Input: part model. Units: mm. Frame: model coordinates. A direction names the side the tool comes from. Coordinates: 2 decimals unless noted, no trailing zeros. Loops run counter-clockwise (first coordinate to the right, second up) from the corner with the lowest first, then second, coordinate; pieces in that order, holes last.
Item 1: Section B-B on x = -115. Return loops of the section in (y, z).
Item 2: Contact query for flat-ended pins moving along their axis: P1, Ø0.5, axis at y = 1, z = -46, coming from the -X side; P2, Ø0.5, axis at x = -48, y = 1, coming from the -Z side; P3, Ø0.8, axis at y = 1, z = -9, coming from the +X side. Output: stop coordinate, or through.
Item 3: Reachability of faces 1 (the flat face through (-176.227, 0.811, -82.597)), 2 (the flat face through (-3.68, 0.81, -83.02)), 3 (the flat face through (-12.056, 0.811, -84.63)), 4 (the flat face through (-91, 1.6, -51)) from +Z, -Z, +X, -X, +Y, -Y: full face, straight path, thin tool, end or side. Return the list, or none.
Item 4: Ray query, line 1 along Z through (x, y) = (-87, 0.6); line 2 along Z through (x, y) = (-103.5, 0.8); line 3 along X through (y, z) = (0.55, -8.5). Return the intervals inside material, ascending.
Item 5: Section D-D on z = -52.5. Return loops of the section in (x, y), and give its area (3 significant figures).
Item 6: Pull-direction query (Z, two-part tool) for faces 5 (the flat face through (-91, 0, -51)), 6 (the flat face through (-175.826, 0.811, -17.954)); classes: released by +Z, released by -Z, zero draft, split by the parting line, or undercut.
Item 7: Section C-C on y = 0.6. Give the number of separate pieces and of enclosed holes in the cut face, and give its area (3 significant figures).
Item 8: Section A-A on z = -109. Return loops of the section in (x, y), and give its area (3 significant figures).
```python
from build123d import *

# Parameters (mm, degrees)
SKETCH1_W           = 80
SKETCH1_H           = 30
SKETCH1_W_2         = 50
BOSS_EXTRUDE1_DEPTH = 1.6
FILLET1_SIZE        = 60
SKETCH6_W           = 80
SKETCH6_H           = 30
CUT_EXTRUDE1_DEPTH  = 10
FILLET3_R           = 20
CUT_EXTRUDE3_REACH  = 256.563
SKETCH9_W           = 15.367
SKETCH9_H           = 16.637
CUT_EXTRUDE5_REACH  = 256.563
SKETCH11_R          = 1.55
SKETCH11_R_2        = 1
SKETCH11_W          = 23.3
SKETCH11_H          = 12.6
CUT_EXTRUDE6_REACH  = 256.563
SKETCH12_W          = 33.087121525
SKETCH12_H          = 10


with BuildPart() as part:
    # Sketch1 → Boss-Extrude1 (new body)
    with BuildSketch(Plane(origin=(0, 0, 0), x_dir=(1, 0, 0), z_dir=(0, 1, 0))):
        with Locations((-90, -15)):
            Rectangle(SKETCH1_W, SKETCH1_H)
        Polygon((0, 180), (-180, 180), (-180, 30), (-130, 30), (-50, 30), (0, 30), align=None)
        with Locations((-25, 15)):
            Rectangle(SKETCH1_W_2, SKETCH1_H)
        with Locations((-155, 15)):
            Rectangle(SKETCH1_W_2, SKETCH1_H)
        with Locations((-90, 15)):
            Rectangle(SKETCH1_W, SKETCH1_H)
    extrude(amount=BOSS_EXTRUDE1_DEPTH)

    # Fillet1
    # a fillet whose section is not a circle: 60 mm, written as the material it takes off along each edge
    with BuildSketch(Plane(origin=(0, -150, -180), x_dir=(0, 0, 1), z_dir=(0, 1, 0)), Plane(origin=(-180, -150, -180), x_dir=(1, 0, 0), z_dir=(0, 1, 0))) as fillet1_piece_1:
        with BuildLine():
            Bezier((FILLET1_SIZE, 0), (0, 0), (0, -FILLET1_SIZE), weights=[1, 0.25, 1])
            Line((0, -FILLET1_SIZE), (0, 0))
            Line((0, 0), (FILLET1_SIZE, 0))
        make_face()
    extrude(amount=301.6, mode=Mode.SUBTRACT)

    # Sketch6 → Cut-Extrude1 (cut)
    with BuildSketch(Plane(origin=(0, 1.6, 0), x_dir=(1, 0, 0), z_dir=(0, 1, 0))):
        with Locations((-90, -15)):
            Rectangle(SKETCH6_W, SKETCH6_H)
        Polygon((-180, 100), (-180, 0), (-173, 30.1112758), (-173, 67.7112758), align=None)
        Polygon((-7, 30.1112758), (0, 0), (0, 100), (-7, 67.7112758), align=None)
    extrude(amount=-CUT_EXTRUDE1_DEPTH, mode=Mode.SUBTRACT)

    # Fillet2
    # a fillet whose section is not a circle: 5 mm, written as the material it takes off along each edge
    with BuildSketch(Plane(origin=(-180, -15.739211431, 0), x_dir=(1, 0, 0), z_dir=(0, 1, 0)), Plane(origin=(0, -15.739211431, 0), x_dir=(-0.22643302171939195, 0, -0.9740267381725335), z_dir=(0, 1, 0))) as fillet2_piece_1:
        with BuildLine():
            Bezier((6.295684572, 0), (0, 0), (1.425550882, 6.132165109), weights=[1, 0.333333333, 1])
            Line((1.425550882, 6.132165109), (0, 0))
            Line((0, 0), (6.295684572, 0))
        make_face()
    extrude(amount=33.078422862, mode=Mode.SUBTRACT)

    # Fillet3
    fillet3_edges = [part.edges().sort_by_distance(p)[0] for p in [
        (0, 0.8, -100),
        (-180, 0.8, -100),
    ]]
    fillet(fillet3_edges, radius=FILLET3_R)

    # Sketch9 → Cut-Extrude3 (cut, up to next)
    with BuildSketch(Plane(origin=(0, 1.6, 0), x_dir=(1, 0, 0), z_dir=(0, 1, 0)), mode=Mode.PRIVATE) as cut_extrude3_sk1:
        Polygon((-164, 113.6), (-164, 67.6), (-16, 67.6), (-8, 102.143047988), (-8, 113.6), align=None)
    cut_extrude3_tool1 = extrude(cut_extrude3_sk1.sketch, amount=-CUT_EXTRUDE3_REACH, mode=Mode.PRIVATE) & part.part
    # Sketch9 → Cut-Extrude3 (cut, up to next)
    with BuildSketch(Plane(origin=(0, 1.6, 0), x_dir=(1, 0, 0), z_dir=(0, 1, 0)), mode=Mode.PRIVATE) as cut_extrude3_sk2:
        with Locations((-90.0575, 134.935)):
            Rectangle(SKETCH9_W, SKETCH9_H)
    cut_extrude3_tool2 = extrude(cut_extrude3_sk2.sketch, amount=-CUT_EXTRUDE3_REACH, mode=Mode.PRIVATE) & part.part
    add(cut_extrude3_tool1.solids().sort_by_distance((-87.479003, 1.6, -90.825495))[0], mode=Mode.SUBTRACT)
    add(cut_extrude3_tool2.solids().sort_by_distance((-90.0575, 1.6, -134.935))[0], mode=Mode.SUBTRACT)

    # Sketch11 → Cut-Extrude5 (cut, up to next)
    with BuildSketch(Plane(origin=(0, 1.6, 0), x_dir=(1, 0, 0), z_dir=(0, 1, 0)), mode=Mode.PRIVATE) as cut_extrude5_sk1:
        with Locations(Location((-170, 9, 0), (0, 0, 270))):
            Circle(SKETCH11_R)
    cut_extrude5_tool1 = extrude(cut_extrude5_sk1.sketch, amount=-CUT_EXTRUDE5_REACH, mode=Mode.PRIVATE) & part.part
    # Sketch11 → Cut-Extrude5 (cut, up to next)
    with BuildSketch(Plane(origin=(0, 1.6, 0), x_dir=(1, 0, 0), z_dir=(0, 1, 0)), mode=Mode.PRIVATE) as cut_extrude5_sk2:
        with Locations(Location((-126.25, 145, 0), (0, 0, 270))):
            Circle(SKETCH11_R)
    cut_extrude5_tool2 = extrude(cut_extrude5_sk2.sketch, amount=-CUT_EXTRUDE5_REACH, mode=Mode.PRIVATE) & part.part
    # Sketch11 → Cut-Extrude5 (cut, up to next)
    with BuildSketch(Plane(origin=(0, 1.6, 0), x_dir=(1, 0, 0), z_dir=(0, 1, 0)), mode=Mode.PRIVATE) as cut_extrude5_sk3:
        with Locations(Location((-10, 9, 0), (0, 0, 270))):
            Circle(SKETCH11_R)
    cut_extrude5_tool3 = extrude(cut_extrude5_sk3.sketch, amount=-CUT_EXTRUDE5_REACH, mode=Mode.PRIVATE) & part.part
    # Sketch11 → Cut-Extrude5 (cut, up to next)
    with BuildSketch(Plane(origin=(0, 1.6, 0), x_dir=(1, 0, 0), z_dir=(0, 1, 0)), mode=Mode.PRIVATE) as cut_extrude5_sk4:
        with Locations(Location((-53.75, 145, 0), (0, 0, 270))):
            Circle(SKETCH11_R)
    cut_extrude5_tool4 = extrude(cut_extrude5_sk4.sketch, amount=-CUT_EXTRUDE5_REACH, mode=Mode.PRIVATE) & part.part
    # Sketch11 → Cut-Extrude5 (cut, up to next)
    with BuildSketch(Plane(origin=(0, 1.6, 0), x_dir=(1, 0, 0), z_dir=(0, 1, 0)), mode=Mode.PRIVATE) as cut_extrude5_sk5:
        with Locations(Location((-32.3, 10, 0), (0, 0, 270))):
            Circle(SKETCH11_R_2)
    cut_extrude5_tool5 = extrude(cut_extrude5_sk5.sketch, amount=-CUT_EXTRUDE5_REACH, mode=Mode.PRIVATE) & part.part
    # Sketch11 → Cut-Extrude5 (cut, up to next)
    with BuildSketch(Plane(origin=(0, 1.6, 0), x_dir=(1, 0, 0), z_dir=(0, 1, 0)), mode=Mode.PRIVATE) as cut_extrude5_sk6:
        with Locations(Location((-59.6, 10, 0), (0, 0, 270))):
            Circle(SKETCH11_R_2)
    cut_extrude5_tool6 = extrude(cut_extrude5_sk6.sketch, amount=-CUT_EXTRUDE5_REACH, mode=Mode.PRIVATE) & part.part
    # Sketch11 → Cut-Extrude5 (cut, up to next)
    with BuildSketch(Plane(origin=(0, 1.6, 0), x_dir=(1, 0, 0), z_dir=(0, 1, 0)), mode=Mode.PRIVATE) as cut_extrude5_sk7:
        with Locations((-45.95, 10)):
            Rectangle(SKETCH11_W, SKETCH11_H)
    cut_extrude5_tool7 = extrude(cut_extrude5_sk7.sketch, amount=-CUT_EXTRUDE5_REACH, mode=Mode.PRIVATE) & part.part
    add(cut_extrude5_tool1.solids().sort_by_distance((-170, 1.6, -9))[0], mode=Mode.SUBTRACT)
    add(cut_extrude5_tool2.solids().sort_by_distance((-126.25, 1.6, -145))[0], mode=Mode.SUBTRACT)
    add(cut_extrude5_tool3.solids().sort_by_distance((-10, 1.6, -9))[0], mode=Mode.SUBTRACT)
    add(cut_extrude5_tool4.solids().sort_by_distance((-53.75, 1.6, -145))[0], mode=Mode.SUBTRACT)
    add(cut_extrude5_tool5.solids().sort_by_distance((-32.3, 1.6, -10))[0], mode=Mode.SUBTRACT)
    add(cut_extrude5_tool6.solids().sort_by_distance((-59.6, 1.6, -10))[0], mode=Mode.SUBTRACT)
    add(cut_extrude5_tool7.solids().sort_by_distance((-45.95, 1.6, -10))[0], mode=Mode.SUBTRACT)

    # Sketch12 → Cut-Extrude6 (cut, up to next)
    with BuildSketch(Plane(origin=(0, 1.6, 0), x_dir=(1, 0, 0), z_dir=(0, 1, 0)), mode=Mode.PRIVATE) as cut_extrude6_sk1:
        with Locations((-90.756439238, 5)):
            Rectangle(SKETCH12_W, SKETCH12_H)
    cut_extrude6_tool1 = extrude(cut_extrude6_sk1.sketch, amount=-CUT_EXTRUDE6_REACH, mode=Mode.PRIVATE) & part.part
    add(cut_extrude6_tool1.solids().sort_by_distance((-90.756439, 1.6, -5))[0], mode=Mode.SUBTRACT)


solid = part.part
```
Results found:
1. outline: (0, -180) - (1.6, -180) - (1.6, -113.6) - (0, -113.6) - close; (0, -67.6) - (1.6, -67.6) - (1.6, 0) - (0, 0) - close
2. P1: stops at x = -173
2. P2: stops at z = -175.56
2. P3: stops at x = -2
3. face 1: -X, +Y, -Y
3. face 2: +X, +Y, -Y
3. face 3: +Y, -Y
3. face 4: +Z, -Z, +X, -X, +Y
4. line 1: z = -180 to -143.25, -126.62 to -113.6, -67.6 to -10
4. line 2: z = -180 to -113.6, -67.6 to -10
4. line 3: x = -178.02 to -171.47, -168.53 to -107.3, -74.21 to -57.6, -34.3 to -11.47, -8.53 to -1.98
5. outline: (-173, 0) - (-7, 0) - (-7, 1.6) - (-173, 1.6) - close
5. area: 266 mm2
6. face 5: zero draft
6. face 6: undercut
7. separate pieces: 1
7. enclosed holes: 9
7. area: 20,900 mm2
8. outline: (-180, 0) - (-164, 0) - (-164, 1.6) - (-180, 1.6) - close; (-8, 0) - (0, 0) - (0, 1.6) - (-8, 1.6) - close
8. area: 38.4 mm2
